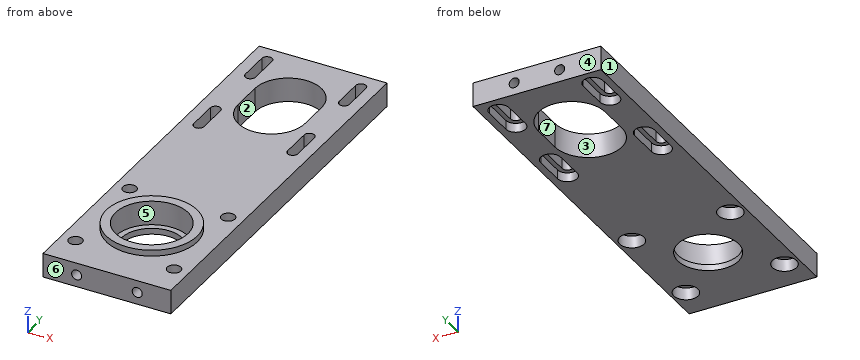
```python
from build123d import *

# Parameters (mm, degrees)
SKETCH_1_W                   = 42.2
SKETCH_1_H                   = 60
EXTRUDE_1_DEPTH              = 4
SKETCH_5_R                   = 15
EXTRUDE_3_DEPTH              = 2
SKETCH_6_R                   = 10
CUT_EXTRUDE_3_DEPTH          = 39.015917719
SKETCH_7_R                   = 12
CUT_EXTRUDE_4_DEPTH          = 8
SKETCH_8_W                   = 42.2
SKETCH_8_H                   = 8
EXTRUDE_4_DEPTH              = 70
CUT_EXTRUDE_5_DEPTH          = 103.689872918
HOLE_START                   = -4
HOLE_WIZARD_M3_7_DEPTH       = 8
HOLE_WIZARD_M3_7_2_DEPTH     = 3
HOLE_WIZARD_M4_1_D           = 4.5
HOLE_WIZARD_M4_1_CBORE_D     = 8
HOLE_WIZARD_M4_1_CBORE_DEPTH = 4
M4X0_7_1_D                   = 3.3
M4X0_7_1_DEPTH               = 10.1
M4X0_7_1_TIP                 = 0.991420021
M4X0_7_2_D                   = 3.3
M4X0_7_2_DEPTH               = 8
M4X0_7_2_TIP                 = 0.991420021


# Read off the part's stored shape, not the designer's step: M3 凹頭蓋螺釘的柱孔7
with BuildPart() as part:
    # 草圖1 → 填料-伸長1 (new, symmetric)
    with BuildSketch(Plane.XY):
        Rectangle(SKETCH_1_W, SKETCH_1_H)
    extrude(amount=EXTRUDE_1_DEPTH, both=True)

    # 草圖5 → 填料-伸長3 (add)
    with BuildSketch(Plane.XY.offset(4)):
        with Locations((0, -3)):
            Circle(SKETCH_5_R)
    extrude(amount=EXTRUDE_3_DEPTH)

    # 草圖6 → 除料-伸長3 (cut, through all)
    with BuildSketch(Plane.XY.offset(6)):
        with Locations((0, -3)):
            Circle(SKETCH_6_R)
    extrude(amount=-CUT_EXTRUDE_3_DEPTH, mode=Mode.SUBTRACT)

    # 草圖7 → 除料-伸長4 (cut)
    with BuildSketch(Plane.XY.offset(6)):
        with Locations((0, -3)):
            Circle(SKETCH_7_R)
    extrude(amount=-CUT_EXTRUDE_4_DEPTH, mode=Mode.SUBTRACT)

    # 草圖8 → 填料-伸長4 (add)
    with BuildSketch(Plane(origin=(0, 30, 0), x_dir=(1, 0, 0), z_dir=(0, 1, 0))):
        Rectangle(SKETCH_8_W, SKETCH_8_H)
    extrude(amount=EXTRUDE_4_DEPTH)

    # 草圖9 → 除料-伸長5 (cut, through all)
    with BuildSketch(Plane(origin=(0, 0, -4), x_dir=(-1, 0, 0), z_dir=(0, 0, -1))):
        with BuildLine():
            Line((11, 79), (11, 69))
            ThreePointArc((11, 69), (0, 58), (-11, 69))
            Line((-11, 69), (-11, 79))
            ThreePointArc((-11, 79), (0, 90), (11, 79))
        make_face()
    extrude(amount=-CUT_EXTRUDE_5_DEPTH, mode=Mode.SUBTRACT)

    # M3 凹頭蓋螺釘的柱孔7 outline → M3 凹頭蓋螺釘的柱孔7 (cut)
    with BuildSketch(Plane.XY.offset(HOLE_START)):
        with BuildLine():
            Line((-13.8, 53.5), (-13.8, 63.5))
            ThreePointArc((-13.8, 63.5), (-15.5, 65.2), (-17.2, 63.5))
            Line((-17.2, 63.5), (-17.2, 53.5))
            ThreePointArc((-17.2, 53.5), (-15.5, 51.8), (-13.8, 53.5))
        make_face()
        with BuildLine():
            Line((-13.8, 84.5), (-13.8, 94.5))
            ThreePointArc((-13.8, 94.5), (-15.5, 96.2), (-17.2, 94.5))
            Line((-17.2, 94.5), (-17.2, 84.5))
            ThreePointArc((-17.2, 84.5), (-15.5, 82.8), (-13.8, 84.5))
        make_face()
        with BuildLine():
            ThreePointArc((17.2, 63.5), (15.5, 65.2), (13.8, 63.5))
            Line((13.8, 63.5), (13.8, 53.5))
            ThreePointArc((13.8, 53.5), (15.5, 51.8), (17.2, 53.5))
            Line((17.2, 53.5), (17.2, 63.5))
        make_face()
        with BuildLine():
            ThreePointArc((17.2, 94.5), (15.5, 96.2), (13.8, 94.5))
            Line((13.8, 94.5), (13.8, 84.5))
            ThreePointArc((13.8, 84.5), (15.5, 82.8), (17.2, 84.5))
            Line((17.2, 84.5), (17.2, 94.5))
        make_face()
    extrude(amount=HOLE_WIZARD_M3_7_DEPTH, mode=Mode.SUBTRACT)

    # Hole Wizard M3 _7 2 outline → Hole Wizard M3 _7 2 (cut)
    # profile 1 of 4: a face of its own
    with BuildSketch(Plane.XY.offset(HOLE_START)):
        with BuildLine():
            ThreePointArc((-12.25, 63.5), (-15.5, 66.75), (-18.75, 63.5))
            Line((-18.75, 63.5), (-18.75, 53.5))
            ThreePointArc((-18.75, 53.5), (-15.5, 50.25), (-12.25, 53.5))
            Line((-12.25, 53.5), (-12.25, 63.5))
        make_face()
        with BuildLine():
            ThreePointArc((-17.2, 63.5), (-15.5, 65.2), (-13.8, 63.5))
            Line((-13.8, 63.5), (-13.8, 53.5))
            ThreePointArc((-13.8, 53.5), (-15.5, 51.8), (-17.2, 53.5))
            Line((-17.2, 53.5), (-17.2, 63.5))
        make_face(mode=Mode.SUBTRACT)
    # profile 2 of 4: a face of its own
    with BuildSketch(Plane.XY.offset(HOLE_START)):
        with BuildLine():
            Line((-12.25, 84.5), (-12.25, 94.5))
            ThreePointArc((-12.25, 94.5), (-15.5, 97.75), (-18.75, 94.5))
            Line((-18.75, 94.5), (-18.75, 84.5))
            ThreePointArc((-18.75, 84.5), (-15.5, 81.25), (-12.25, 84.5))
        make_face()
        with BuildLine():
            ThreePointArc((-17.2, 94.5), (-15.5, 96.2), (-13.8, 94.5))
            Line((-13.8, 94.5), (-13.8, 84.5))
            ThreePointArc((-13.8, 84.5), (-15.5, 82.8), (-17.2, 84.5))
            Line((-17.2, 84.5), (-17.2, 94.5))
        make_face(mode=Mode.SUBTRACT)
    # profile 3 of 4: a face of its own
    with BuildSketch(Plane.XY.offset(HOLE_START)):
        with BuildLine():
            ThreePointArc((18.75, 63.5), (15.5, 66.75), (12.25, 63.5))
            Line((12.25, 63.5), (12.25, 53.5))
            ThreePointArc((12.25, 53.5), (15.5, 50.25), (18.75, 53.5))
            Line((18.75, 53.5), (18.75, 63.5))
        make_face()
        with BuildLine():
            Line((13.8, 53.5), (13.8, 63.5))
            ThreePointArc((13.8, 63.5), (15.5, 65.2), (17.2, 63.5))
            Line((17.2, 63.5), (17.2, 53.5))
            ThreePointArc((17.2, 53.5), (15.5, 51.8), (13.8, 53.5))
        make_face(mode=Mode.SUBTRACT)
    # profile 4 of 4: a face of its own
    with BuildSketch(Plane.XY.offset(HOLE_START)):
        with BuildLine():
            Line((18.75, 84.5), (18.75, 94.5))
            ThreePointArc((18.75, 94.5), (15.5, 97.75), (12.25, 94.5))
            Line((12.25, 94.5), (12.25, 84.5))
            ThreePointArc((12.25, 84.5), (15.5, 81.25), (18.75, 84.5))
        make_face()
        with BuildLine():
            Line((13.8, 84.5), (13.8, 94.5))
            ThreePointArc((13.8, 94.5), (15.5, 96.2), (17.2, 94.5))
            Line((17.2, 94.5), (17.2, 84.5))
            ThreePointArc((17.2, 84.5), (15.5, 82.8), (13.8, 84.5))
        make_face(mode=Mode.SUBTRACT)
    extrude(amount=HOLE_WIZARD_M3_7_2_DEPTH, mode=Mode.SUBTRACT)

    # M4 凹頭蓋螺釘的柱孔1 (through all)
    with Locations(Plane(origin=(0, 0, -4), x_dir=(-1, 0, 0), z_dir=(0, 0, -1))):
        with Locations((16.263455967, 13.263455967), (-16.263455967, -19.263455967), (-16.263455967, 13.263455967), (16.263455967, -19.263455967)):
            CounterBoreHole(HOLE_WIZARD_M4_1_D / 2, HOLE_WIZARD_M4_1_CBORE_D / 2, HOLE_WIZARD_M4_1_CBORE_DEPTH)

    # M4x0.7 螺紋孔1
    with Locations(Plane(origin=(0, -30, 0), x_dir=(-1, 0, 0), z_dir=(0, -1, 0))):
        with Locations((10, 0), (-10, 0)):
            Hole(M4X0_7_1_D / 2, depth=M4X0_7_1_DEPTH)
            with Locations((0, 0, -(M4X0_7_1_DEPTH + M4X0_7_1_TIP / 2))):  # 118° drill point
                Cone(0, M4X0_7_1_D / 2, M4X0_7_1_TIP, mode=Mode.SUBTRACT)

    # M4x0.7 螺紋孔2
    with Locations(Plane(origin=(0, 100, 0), x_dir=(1, 0, 0), z_dir=(0, 1, 0))):
        with Locations((-7.5, 0), (7.5, 0)):
            Hole(M4X0_7_2_D / 2, depth=M4X0_7_2_DEPTH)
            with Locations((0, 0, -(M4X0_7_2_DEPTH + M4X0_7_2_TIP / 2))):  # 118° drill point
                Cone(0, M4X0_7_2_D / 2, M4X0_7_2_TIP, mode=Mode.SUBTRACT)


solid = part.part
```
The model under review builds one solid part; all positions refer to its coordinate system, in mm. Face numbers are marked on the shaded views. A direction names the side the tool comes from. Give positions to 0.01 mm unless a question says otherwise; leave off trailing zeros. Write each loop counter-clockwise with the first axis right and the second up, starting at its lowest first coordinate (ties: lowest second). Pieces come first, ordered by that corner, then holes.
(1) The part is to be moulded in two halves that separate along X. For the marked faces 1, 2, 3 and 4, say which applies: released by +X, released by -X, zero draft, split by the parting line, or undercut.
(2) To check wall thickness, follow L1, parallel to Y at x = 0, z = -2.9; L2, parallel to X at y = -3.5, z = 0.5; L3, parallel to Y at x = -17, z = -2. State the ranges of each line that lie inside material, in increasing order.
(3) Consider section B-B, the plane x = -3.5. Give the boundary of the cut face in (y, z), and give its area (3 significant figures).
(4) Consider section D-D, the plane x = 3. Give the boundary of the cut face in (y, z).
(5) Consider section A-A, the plane y = 71. Give the boundary of the cut face in (x, z).
(6) Consider section C-C, the plane y = 3. Give the boundary of the cut face in (x, z).
(7) Tool access review of the marked faces 5, 6 and 7: name each direction out of +Z, -Z, +X, -X, +Y, -Y from which nothing blocks a thin tool from reaching the whole face with its end or side.
(8) For P1, Ø14.5, axis at x = 0, y = -3, coming from the -Z side; P2, Ø6, axis at x = 16.26, y = -19.26, coming from the +Z side; P3, Ø3, axis at x = -14, y = 60, coming from the -Z side; P4, Ø4, axis at x = 16.5, z = 4.5, coming from the +Y side, all flat-tipped, find the tip position at first contact; note any pin that passes through.
Returned:
1. face 1: released by -X
1. face 2: undercut
1. face 3: undercut
1. face 4: zero draft
2. L1: y = -30 to -13, 7 to 58, 90 to 100
2. L2: x = -21.1 to -11.99, 11.99 to 21.1
2. L3: y = -30 to -23.2, -15.33 to 9.33, 17.2 to 50.62, 66.38 to 81.62, 97.38 to 100
3. outline: (-30, -4) - (-12.37, -4) - (-12.37, -2) - (-14.48, -2) - (-14.48, 6) - (-17.59, 6) - (-17.59, 4) - (-30, 4) - close; (6.37, -4) - (58.57, -4) - (58.57, 4) - (11.59, 4) - (11.59, 6) - (8.48, 6) - (8.48, -2) - (6.37, -2) - close; (89.43, -4) - (100, -4) - (100, 4) - (89.43, 4) - close
3. area: 630 mm2
4. outline: (-30, -4) - (-12.54, -4) - (-12.54, -2) - (-14.62, -2) - (-14.62, 6) - (-17.7, 6) - (-17.7, 4) - (-30, 4) - close; (6.54, -4) - (58.42, -4) - (58.42, 4) - (11.7, 4) - (11.7, 6) - (8.62, 6) - (8.62, -2) - (6.54, -2) - close; (89.58, -4) - (100, -4) - (100, 4) - (89.58, 4) - close
5. outline: (-21.1, -4) - (-11, -4) - (-11, 4) - (-21.1, 4) - close; (11, -4) - (21.1, -4) - (21.1, 4) - (11, 4) - close
6. outline: (-21.1, -4) - (-8, -4) - (-8, -2) - (-10.39, -2) - (-10.39, 6) - (-13.75, 6) - (-13.75, 4) - (-21.1, 4) - close; (8, -4) - (21.1, -4) - (21.1, 4) - (13.75, 4) - (13.75, 6) - (10.39, 6) - (10.39, -2) - (8, -2) - close
7. face 5: +Z
7. face 6: +Z, -Z, +X, -X, -Y
7. face 7: +Z, -Z
8. P1: passes through
8. P2: stops at z = 4
8. P3: stops at z = -1
8. P4: stops at y = 100
